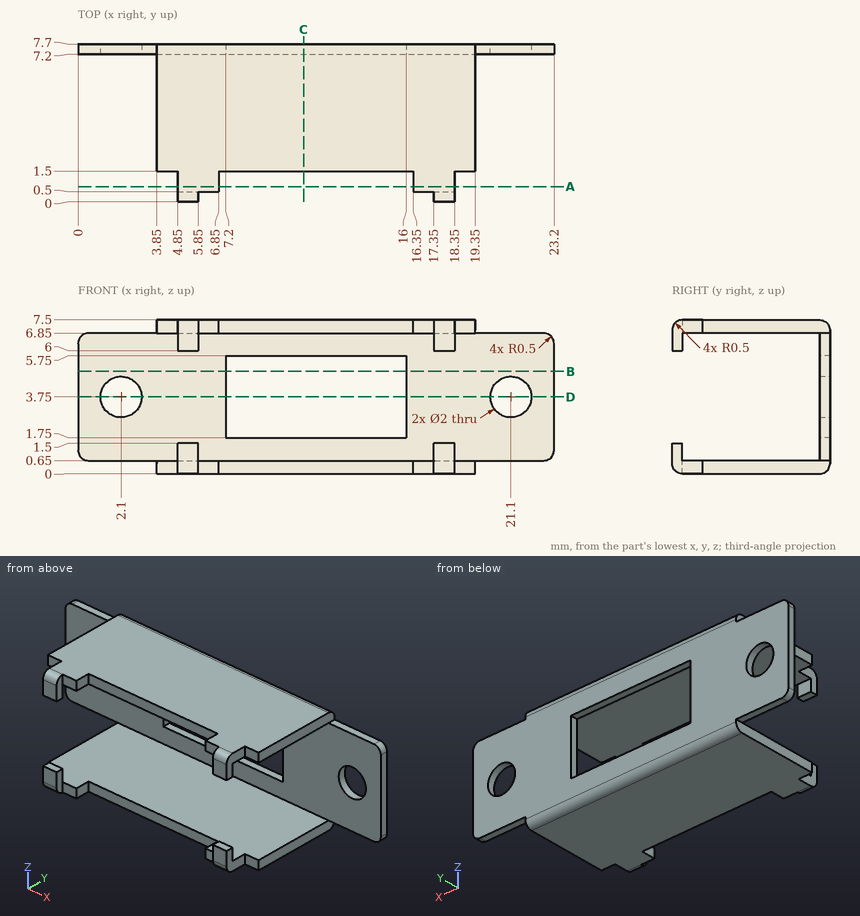
Drawing for the job (mm, zero at the part's lowest x, y, z). Give positions to 0.01 mm unless a question says otherwise; leave off trailing zeros. Order: outer loops, then holes, each group sorted by start corner. A loop starts at its lowest first (then second) coordinate and runs counter-clockwise, first axis right, second up. Notation, with made-up numbers: (41.25, 74.25) - (87.25, 74.25) arc R18 cw to (87.25, 96.25) - close; hole circle Ø7 at (-20, -15). An arc over 180 degrees is marked (long way). Write item = value, one per line. Start each with the question number.
1. Cut at C-C, the plane x = 11. List the corners of the cut face in (y, z), and give its area (3 significant figures).
2. Cut at A-A, the plane y = 0.75. List the corners of the cut face in (x, z), and give its area (3 significant figures).
3. Cut at D-D, the plane z = 3.75. List the corners of the cut face in (x, y), and give its area (3 significant figures).
4. Cut at B-B, the plane z = 5. List the corners of the cut face in (x, y).
5. Drop flat-ended pins along their axis: P1, Ø3, axis at y = 6.5, z = 3, coming from the +X side; P2, Ø0.5, axis at y = 1, z = 7, coming from the -X side; P3, Ø0.7, axis at x = 6.5, z = 7, coming from the -Y side; P4, Ø4, axis at y = 4, z = 2.5, coming from the -X side. Give the stop position or say it passes through.
6. Probe line 1 along X through (y, z) = (7.5, 3.75); line 2 along Y through (x, z) = (5.25, 6.5); line 3 along Z through (x, y) = (15.75, 7). List the from-to ranges inside material, lowest first.
Taken from the geometry:
q1.outline = (1.5, 0) - (7.2, 0) arc R0.5 ccw to (7.7, 0.5) - (7.7, 1.75) - (7.2, 1.75) - (7.2, 0.65) - (1.5, 0.65) - close; (1.5, 6.85) - (7.2, 6.85) - (7.2, 5.75) - (7.7, 5.75) - (7.7, 7) arc R0.5 ccw to (7.2, 7.5) - (1.5, 7.5) - close
q1.area = 9.05 mm²
q2.outline = (4.85, 0) - (6.85, 0) - (6.85, 0.65) - (4.85, 0.65) - close; (4.85, 6.85) - (6.85, 6.85) - (6.85, 7.5) - (4.85, 7.5) - close; (16.35, 0) - (18.35, 0) - (18.35, 0.65) - (16.35, 0.65) - close; (16.35, 6.85) - (18.35, 6.85) - (18.35, 7.5) - (16.35, 7.5) - close
q2.area = 5.20 mm²
q3.outline = (0, 7.2) - (1.1, 7.2) - (1.1, 7.7) - (0, 7.7) - close; (3.1, 7.2) - (7.2, 7.2) - (7.2, 7.7) - (3.1, 7.7) - close; (16, 7.2) - (20.1, 7.2) - (20.1, 7.7) - (16, 7.7) - close; (22.1, 7.2) - (23.2, 7.2) - (23.2, 7.7) - (22.1, 7.7) - close
q3.area = 5.20 mm²
q4.outline = (0, 7.2) - (7.2, 7.2) - (7.2, 7.7) - (0, 7.7) - close; (16, 7.2) - (23.2, 7.2) - (23.2, 7.7) - (16, 7.7) - close
q5.P1 = 23.2
q5.P2 = 4.85
q5.P3 = 0.5
q5.P4 = 3.85
q6.line_1 = 0 to 1.1, 3.1 to 7.2, 16 to 20.1, 22.1 to 23.2
q6.line_2 = 0 to 0.5, 7.2 to 7.7
q6.line_3 = 0 to 0.65, 6.85 to 7.5
